The listing builds one solid part. Answer for the finished solid, in the listing's coordinates (mm). Round coordinates to 2 decimals unless told otherwise and drop trailing zeros. Write each loop counter-clockwise with the first axis right and the second up, starting at its lowest first coordinate (ties: lowest second). Pieces come first, ordered by that corner, then holes.
from build123d import *

# Parameters (mm, degrees)
SKETCH1_R           = 15
SKETCH1_R_2         = 1.65
SKETCH1_R_3         = 2.65
SKETCH1_R_4         = 1.1
BOSS_EXTRUDE1_DEPTH = 1.5
CUT_EXTRUDE1_START  = 1
SKETCH1_5_R         = 1.65
SKETCH1_5_R_2       = 1.1
CUT_EXTRUDE1_DEPTH  = 0.5


with BuildPart() as part:
    # Sketch1 → Boss-Extrude1 (new body)
    # profile 1 of 4: a face of its own
    with BuildSketch(Plane.XY):
        Circle(SKETCH1_R)
        with Locations((-9.526279442, -5.5)):
            Circle(SKETCH1_R_2, mode=Mode.SUBTRACT)
        with Locations((9.526279442, -5.5)):
            Circle(SKETCH1_R_2, mode=Mode.SUBTRACT)
        with Locations((0, 11)):
            Circle(SKETCH1_R_2, mode=Mode.SUBTRACT)
        with Locations((-9.959292144, 5.75)):
            Circle(SKETCH1_R_3, mode=Mode.SUBTRACT)
        with Locations((0, -11.5)):
            Circle(SKETCH1_R_3, mode=Mode.SUBTRACT)
        with Locations((9.959292144, 5.75)):
            Circle(SKETCH1_R_3, mode=Mode.SUBTRACT)
    # profile 2 of 4: a face of its own
    with BuildSketch(Plane.XY):
        with Locations((9.526279442, -5.5)):
            Circle(SKETCH1_R_2)
        with Locations((9.526279442, -5.5)):
            Circle(SKETCH1_R_4, mode=Mode.SUBTRACT)
    # profile 3 of 4: a face of its own
    with BuildSketch(Plane.XY):
        with Locations((0, 11)):
            Circle(SKETCH1_R_2)
        with Locations((0, 11)):
            Circle(SKETCH1_R_4, mode=Mode.SUBTRACT)
    # profile 4 of 4: a face of its own
    with BuildSketch(Plane.XY):
        with Locations((-9.526279442, -5.5)):
            Circle(SKETCH1_R_2)
        with Locations((-9.526279442, -5.5)):
            Circle(SKETCH1_R_4, mode=Mode.SUBTRACT)
    extrude(amount=BOSS_EXTRUDE1_DEPTH)

    # Sketch1<5> → Cut-Extrude1 (cut)
    # profile 1 of 3: a face of its own
    with BuildSketch(Plane.XY.offset(CUT_EXTRUDE1_START)):
        with Locations((-9.526279442, -5.5)):
            Circle(SKETCH1_5_R)
        with Locations((-9.526279442, -5.5)):
            Circle(SKETCH1_5_R_2, mode=Mode.SUBTRACT)
    # profile 2 of 3: a face of its own
    with BuildSketch(Plane.XY.offset(CUT_EXTRUDE1_START)):
        with Locations((0, 11)):
            Circle(SKETCH1_5_R)
        with Locations((0, 11)):
            Circle(SKETCH1_5_R_2, mode=Mode.SUBTRACT)
    # profile 3 of 3: a face of its own
    with BuildSketch(Plane.XY.offset(CUT_EXTRUDE1_START)):
        with Locations((9.526279442, -5.5)):
            Circle(SKETCH1_5_R)
    extrude(amount=CUT_EXTRUDE1_DEPTH, mode=Mode.SUBTRACT)


solid = part.part
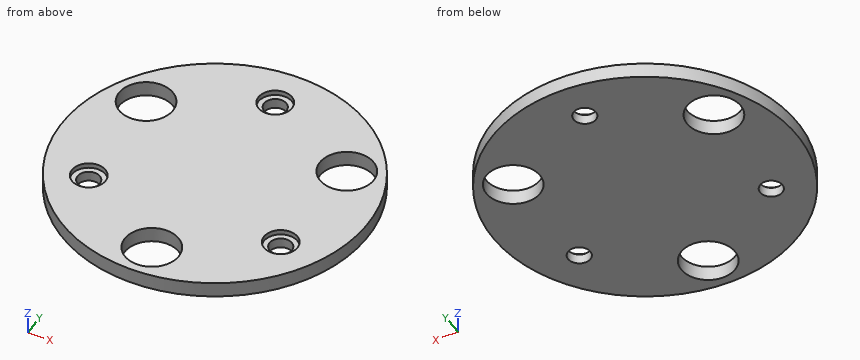
1. Section A-A on x = 0 is taken. Determine the outline of the cut face in (y, z).
Geometry says:
outline: (-15, 0) - (-14.15, 0) - (-14.15, 1.5) - (-15, 1.5) - close; (-8.85, 0) - (9.9, 0) - (9.9, 1) - (9.35, 1) - (9.35, 1.5) - (-8.85, 1.5) - close; (12.1, 0) - (15, 0) - (15, 1.5) - (12.65, 1.5) - (12.65, 1) - (12.1, 1) - close
2. Section C-C on y = -11.5 is taken. Determine the outline of the cut face in (x, z), plus the area to 3 significant figures.
Geometry says:
outline: (-9.63, 0) - (-2.65, 0) - (-2.65, 1.5) - (-9.63, 1.5) - close; (2.65, 0) - (9.63, 0) - (9.63, 1.5) - (2.65, 1.5) - close
area: 20.9 mm2
3. Section B-B on z = 0.7 is taken. Determine the outline of the cut face in (x, y), plus the area to 3 significant figures.
Geometry says:
outline: circle Ø30 at (0, 0); hole circle Ø5.3 at (-9.96, 5.75); hole circle Ø2.2 at (-9.53, -5.5); hole circle Ø5.3 at (0, -11.5); hole circle Ø2.2 at (0, 11); hole circle Ø5.3 at (9.96, 5.75); hole circle Ø2.2 at (9.53, -5.5)
area: 629 mm2
4. Straight lines are drawn through the part: line 1 along Y through (x, z) = (0, 1.35); line 2 along Y through (x, z) = (0.75, 0.8); line 3 along X through (y, z) = (-4.5, 1.4). For each, find the intervals that lie inside material, in ascending order.
Geometry says:
line 1: y = -15 to -14.15, -8.85 to 9.35, 12.65 to 15
line 2: y = -14.98 to -14.04, -8.96 to 10.2, 11.8 to 14.98
line 3: x = -14.31 to -10.84, -8.21 to 8.21, 10.84 to 14.31
5. Given pin 1 (2 mm diameter, centred on x = 9.53, y = -5.5, fed in from +Z); pin 2 (4.5 mm diameter, centred on x = 0, y = 11, fed in from -Z); pin 3 (3 mm diameter, centred on x = 0, y = 11, fed in from +Z), each flat-ended and moving along its own axis, determine where each tip first touches the part or whether it passes through.
Geometry says:
pin 1: passes through
pin 2: stops at z = 0
pin 3: stops at z = 1
6. Section D-D on y = 5.75 is taken. Determine the outline of the cut face in (x, z), plus the area to 3 significant figures.
Geometry says:
outline: (-13.85, 0) - (-12.61, 0) - (-12.61, 1.5) - (-13.85, 1.5) - close; (-7.31, 0) - (7.31, 0) - (7.31, 1.5) - (-7.31, 1.5) - close; (12.61, 0) - (13.85, 0) - (13.85, 1.5) - (12.61, 1.5) - close
area: 25.7 mm2
